```python
from build123d import *

# Parameters (mm, degrees)
F1_DEPTH = 240
F2_R     = 15
F3_R     = 10
F5_DEPTH = 10
F7_DEPTH = 10
F8_R     = 5
F9_R     = 5
F10_R    = 5


with BuildPart() as f1:
    # F0 (on Front) → F1 (new body)
    with BuildSketch(Plane.XZ):
        Polygon((-22.5, -22.5), (22.5, -22.5), (22.5, 22.5), (2.5, 22.5), (2.5, -2.5), (-22.5, -2.5), align=None)
    extrude(amount=F1_DEPTH)

    # F2
    f2_edges = [f1.edges().sort_by_distance(p)[0] for p in [
        (2.5, -120, -2.5),
    ]]
    fillet(f2_edges, radius=F2_R)

    # F3
    f3_edges = [f1.edges().sort_by_distance(p)[0] for p in [
        (22.5, -120, -22.5),
    ]]
    fillet(f3_edges, radius=F3_R)

    # F4 (on face) → F5 (cut)
    with BuildSketch(Plane.XY.offset(22.5)):
        with BuildLine():
            Line((7.5, -15), (7.5, -225))
            ThreePointArc((7.5, -225), (12.5, -230), (17.5, -225))
            Line((17.5, -225), (17.5, -15))
            ThreePointArc((17.5, -15), (12.5, -10), (7.5, -15))
        make_face()
    extrude(amount=-F5_DEPTH, mode=Mode.SUBTRACT)

    # F6 (on face) → F7 (cut)
    with BuildSketch(Plane(origin=(-22.5, 0, 0), x_dir=(0, -1, 0), z_dir=(-1, 0, 0))):
        with BuildLine():
            Line((225, -7.5), (15, -7.5))
            ThreePointArc((15, -7.5), (10, -12.5), (15, -17.5))
            Line((15, -17.5), (225, -17.5))
            ThreePointArc((225, -17.5), (230, -12.5), (225, -7.5))
        make_face()
    extrude(amount=-F7_DEPTH, mode=Mode.SUBTRACT)

    # F8
    f8_edges = [f1.edges().sort_by_distance(p)[0] for p in [
        (22.5, -240, 5),
        (19.571068, -240, -19.571068),
    ]]
    fillet(f8_edges, radius=F8_R)

    # F9
    f9_edges = [f1.edges().sort_by_distance(p)[0] for p in [
        (22.5, 0, 5),
    ]]
    fillet(f9_edges, radius=F9_R)

    # F10
    f10_edges = [f1.edges().sort_by_distance(p)[0] for p in [
        (-1.893398, -240, 1.893398),
        (-1.893398, 0, 1.893398),
    ]]
    fillet(f10_edges, radius=F10_R)


solid = f1.part
```
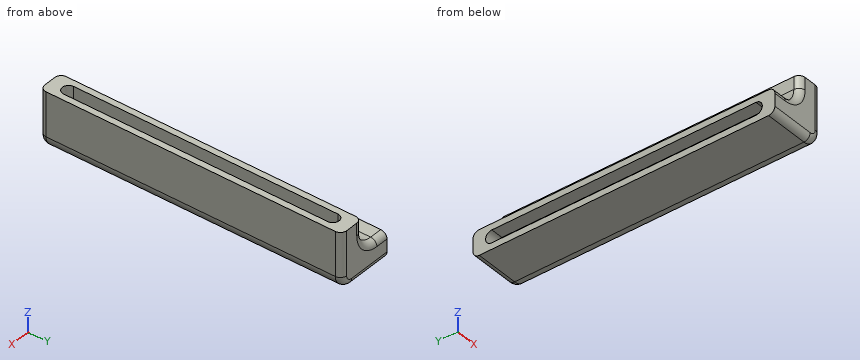
For this review, take the finished solid that the model builds, in its own axes (mm). Coordinates: 2 decimals unless noted, no trailing zeros. Write each loop counter-clockwise with the first axis right and the second up, starting at its lowest first coordinate (ties: lowest second). Pieces come first, ordered by that corner, then holes. Notation, with made-up numbers: (69, 28.25) - (108, 28.25) arc R22 cw to (108, 66.25) - close; hole circle Ø1 at (27.5, -23.75). An arc over 180 degrees is marked (long way). Answer in a Markdown table with one row per item. Add a question column.
Q1. For P1, Ø11, axis at y = -75, z = -13, coming from the -X side; P2, Ø3, axis at x = -19, y = -129, coming from the +Z side; P3, Ø5, axis at y = -166, z = 17, coming from the -X side; P4, Ø4, axis at y = -56, z = -12, coming from the -X side, all flat-tipped, find the tip position at first contact; note any pin that passes through.
Q2. For probe 1 along Z at (x, y) = (-19.5, -205); probe 2 along X at (y, z) = (-132, 19); probe 3 along Z at (x, y) = (9.5, -123), list the stretches that pass through material, from the lowest coordinate up.
Q3. We need section B-B, the plane y = -210.5. State the section outline as (x, z) points.
Q4. We need section A-A, the plane z = 19.5. State the section outline as (x, y) points.
Answer list:
| question | item | result |
|---|---|---|
| 1 | P1 | stops at x = -22.5 |
| 1 | P2 | stops at z = -2.5 |
| 1 | P3 | stops at x = 2.5 |
| 1 | P4 | stops at x = -12.5 |
| 2 | probe 1 | z = -22.5 to -17.5, -7.5 to -2.5 |
| 2 | probe 2 | x = 2.5 to 7.5, 17.5 to 22.5 |
| 2 | probe 3 | z = -22.5 to 12.5 |
| 3 | outline | (-22.5, -22.5) - (12.5, -22.5) arc R10 ccw to (22.5, -12.5) - (22.5, 22.5) - (17.5, 22.5) - (17.5, 12.5) - (7.5, 12.5) - (7.5, 22.5) - (2.5, 22.5) - (2.5, 12.5) arc R15 cw to (-12.5, -2.5) - (-22.5, -2.5) - (-22.5, -7.5) - (-12.5, -7.5) - (-12.5, -17.5) - (-22.5, -17.5) - close |
| 4 | outline | (2.5, -235) arc R5 ccw to (7.5, -240) - (17.5, -240) arc R5 ccw to (22.5, -235) - (22.5, -5) arc R5 ccw to (17.5, 0) - (7.5, 0) arc R5 ccw to (2.5, -5) - close; hole (7.5, -225) arc R5 ccw to (17.5, -225) - (17.5, -15) arc R5 ccw to (7.5, -15) - close |
